Could you check a few things on this drawing? It's one solid part, dimensions in mm from its lowest x, y, z. Give positions to 0.01 mm unless a question says otherwise; leave off trailing zeros. Order: outer loops, then holes, each group sorted by start corner. A loop starts at its lowest first (then second) coordinate and runs counter-clockwise, first axis right, second up. Notation, with made-up numbers: M 25.5,5.5 L 56.5,5.5 A22 cw 56.5,19.5 Z; hole C 78.25,81 d3. An arc over 180 degrees is marked long. Return JSON: item names as keys, results as strings. Group by question number.
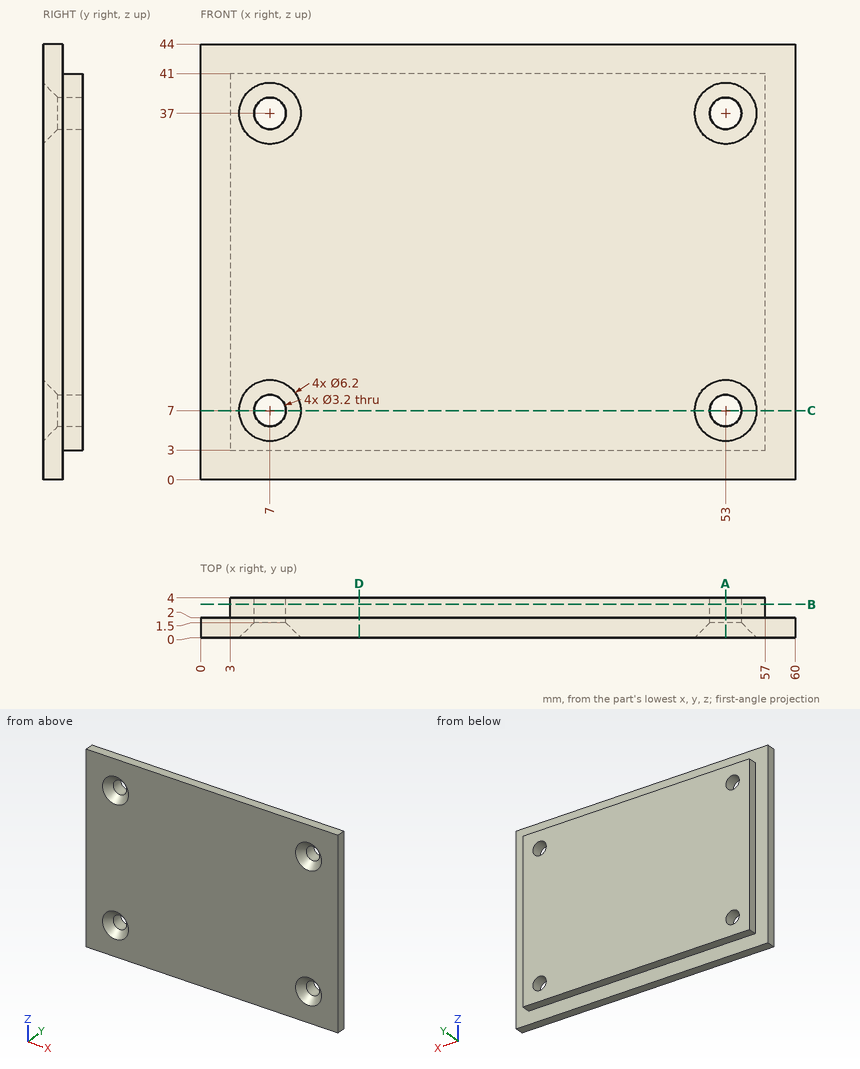
1. Imagine slicing it at D-D, the plane x = 16. Please give me the cut outline in (y, z), plus the area to 3 significant figures.
2. Imagine slicing it at A-A, the plane x = 53. Please give me the cut outline in (y, z).
3. Imagine slicing it at B-B, the plane y = 3.35. Please give me the cut outline in (x, z), plus the area to 3 significant figures.
4. Imagine slicing it at C-C, the plane z = 7. Please give me the cut outline in (x, y), plus the area to 3 significant figures.
5. I need wall thicknesses on L1, parallel to X at y = 3.4, z = 37; L2, parallel to Z at x = 7, y = 2.95; L3, parallel to Z at x = 55, y = 2.1. Which ranges of each line are inside material? Lowest first, please. Write a range as from..to.
6. For pin 1 (0.6 mm diameter, centred on x = 40, y = 3.5, fed in from +Z); pin 2 (2 mm diameter, centred on y = 3.5, z = 22, fed in from -X); pin 3 (1.6 mm diameter, centred on x = 28, y = 3.5, fed in from -Z); pin 4 (3 mm diameter, centred on x = 53, z = 37, fed in from +Y), each with a flat end and sliding along its axis, tell me the tip position at first contact or that it passes through.
Values:
{
 "1": {"outline": "M 0,0 L 2,0 L 2,3 L 4,3 L 4,41 L 2,41 L 2,44 L 0,44 Z", "area": "164 mm²"},
 "2": {"outline": "M 0,0 L 2,0 L 2,3 L 4,3 L 4,5.4 L 1.5,5.4 L 0,3.9 Z; M 0,10.1 L 1.5,8.6 L 4,8.6 L 4,35.4 L 1.5,35.4 L 0,33.9 Z; M 0,40.1 L 1.5,38.6 L 4,38.6 L 4,41 L 2,41 L 2,44 L 0,44 Z"},
 "3": {"outline": "M 3,3 L 57,3 L 57,41 L 3,41 Z; hole C 7,7 d3.2; hole C 7,37 d3.2; hole C 53,7 d3.2; hole C 53,37 d3.2", "area": "2,020 mm²"},
 "4": {"outline": "M 0,0 L 3.9,0 L 5.4,1.5 L 5.4,4 L 3,4 L 3,2 L 0,2 Z; M 8.6,1.5 L 10.1,0 L 49.9,0 L 51.4,1.5 L 51.4,4 L 8.6,4 Z; M 54.6,1.5 L 56.1,0 L 60,0 L 60,2 L 57,2 L 57,4 L 54.6,4 Z", "area": "198 mm²"},
 "5": {"L1": "x = 3..5.4, 8.6..51.4, 54.6..57", "L2": "z = 3..5.4, 8.6..35.4, 38.6..41", "L3": "z = 3..41"},
 "6": {"pin 1": "stops at z = 41", "pin 2": "stops at x = 3", "pin 3": "stops at z = 3", "pin 4": "passes through"}
}
